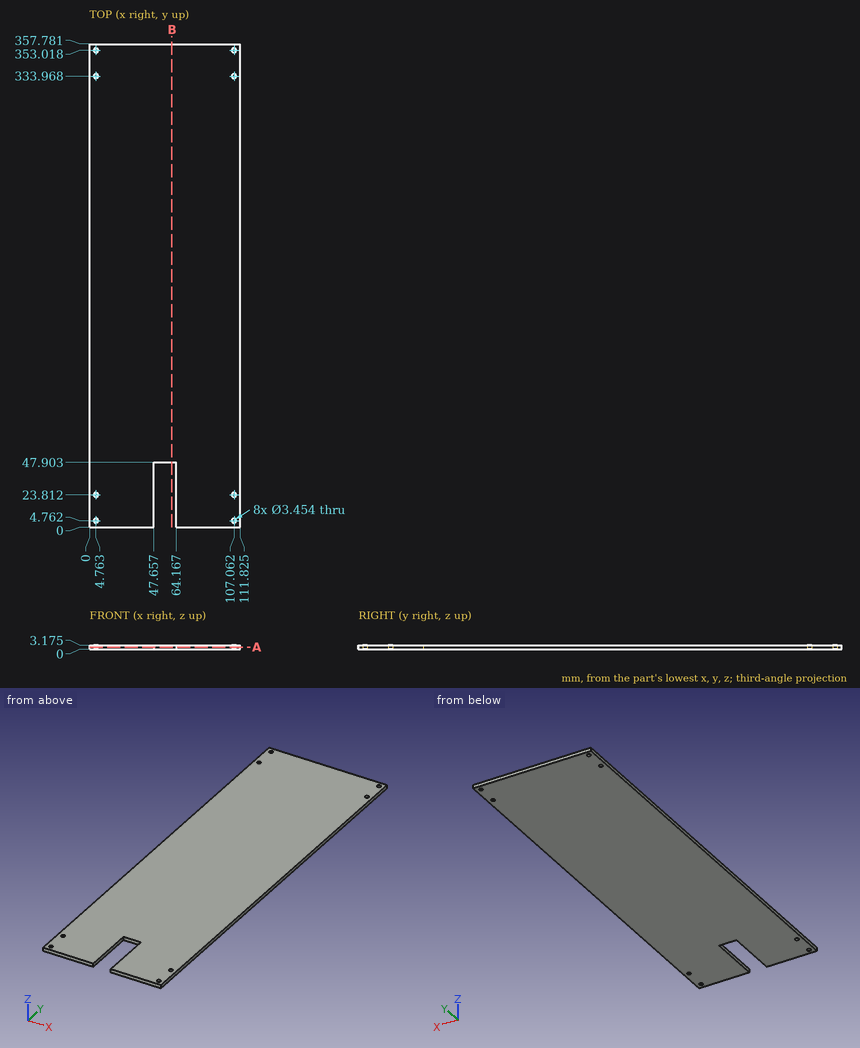
Part print with two shaded views. Sizes in mm from the minimum x, y, z corner. Round coordinates to 2 decimals unless told otherwise and drop trailing zeros. Order: outer loops, then holes, each group sorted by start corner. A loop starts at its lowest first (then second) coordinate and runs counter-clockwise, first axis right, second up. Notation, with made-up numbers: (29.25, 81) -> (73.25, 81) arc R17 ccw to (73.25, 114) -> close; hole circle Ø2 at (21.5, -36.75). An arc over 180 degrees is marked (long way). Use one line per item in the form item = value.
Item 1: Cut at A-A, the plane z = 1.6. Give the number of separate pieces and of enclosed holes in the cut face, and give its area (3 significant figures).
Returned:
separate_pieces = 1
enclosed_holes = 8
area = 39,100 mm^2
Item 2: Drill centre lines: line 1 (X direction, y = 31, z = 0.4) (1 decimal); line 2 (Y direction, x = 60.5, z = 0.35). Where is each one in solid material? Low to high.
Returned:
line_1 = 0 to 47.7, 64.2 to 111.8
line_2 = 47.9 to 357.78
Item 3: Cut at B-B, the plane x = 61. Write the cut outline in (y, z) (1 decimal).
Returned:
outline = (47.9, 0) -> (357.8, 0) -> (357.8, 3.2) -> (47.9, 3.2) -> close
Item 4: Flat gauge pin, fed straight in: pin 1 Ø1 at (x, z) = (55.5, 2) entering from -Y. Where does the tip first touch, or does it go through?
Returned:
pin_1 = 47.9
